Work out the finished part from the listing and answer in its coordinate system (mm). A direction names the side the tool comes from. Coordinates: 2 decimals unless noted, no trailing zeros. Order: outer loops, then holes, each group sorted by start corner. A loop starts at its lowest first (then second) coordinate and runs counter-clockwise, first axis right, second up. Notation, with made-up numbers: (47.25, 72) -> (94.25, 72) arc R21 cw to (94.25, 91) -> close; hole circle Ø1 at (73.25, 22.5). An arc over 180 degrees is marked (long way). Write item = value, one per line. Start each with the question number.
Q1. The part is cut by section A-A, the plane y = 0. Determine the outline of the cut face in (x, z).
Q2. The part is cut by section B-B, the plane z = 0. Determine the outline of the cut face in (x, y).
Q3. Straight lines are drawn through the part: L1, parallel to Z at x = 4.25, y = 0; L2, parallel to X at y = 44, z = 3; L3, parallel to Z at x = 5, y = -44.45. For each, find the intervals that lie inside material, in ascending order. Write a range as from..to.
Q4. Flat-ended cylindrical pins translate along their axes: pin 1 (1 mm diameter, centred on x = 1, y = 7.5, fed in from +Z); pin 2 (5 mm diameter, centred on y = 11, z = 8, fed in from -X); pin 3 (8 mm diameter, centred on y = -16.5, z = -25.5, fed in from -X); pin 4 (1.9 mm diameter, centred on y = 0, z = 44.45, fed in from -X). Find the tip coordinate at first contact, or state that the pin passes through.
Q5. Which of the six approach directions +Z, -Z, +X, -X, +Y, -Y give full straight-line access (tool end or side, diameter ignored) to faces 4 (the cylindrical face through (-7.764, 2.477, -11.155)), 5 (the cylindrical face through (6.26, 0.34, 42.9))?
Q6. The part is cut by section C-C, the plane x = 2. Count the separate pieces of the cut face and the enclosed holes in it, plus the area to 3 significant figures.
Q7. The part is cut by section D-D, the plane y = -44.45. Determine the outline of the cut face in (x, z).
Q8. For a pull along Y with two mould halves and no side action, classify faces 1 (the cylindrical face through (6.3, -10.5, -47.3)), 2 (the flat face through (-15.748, 0, 0)), 3 (the cylindrical face through (6.261, 46.036, 0.07)) as +Y half, -Y half, draft (parallel to the pull), parting line (faces both ways), or undercut.
```python
from build123d import *

# Parameters (mm, degrees)
F0_R     = 48.449945
F1_DEPTH = 12.7
F2_R     = 11.427041
F3_DEPTH = 15.748
F4_R     = 1.5875
F4_R_2   = 1.71099
F5_DEPTH = 12.7


with BuildPart() as f1:
    # F0 (on Right) → F1 (new body)
    with BuildSketch(Plane.YZ):
        Circle(F0_R)
    extrude(amount=F1_DEPTH)

    # F2 (on face) → F3 (join)
    with BuildSketch(Plane(origin=(0, 0, 0), x_dir=(0, -1, 0), z_dir=(-1, 0, 0))):
        Circle(F2_R)
    extrude(amount=F3_DEPTH)

    # F4 (on face) → F5 (cut)
    with BuildSketch(Plane(origin=(0, 0, 0), x_dir=(0, -1, 0), z_dir=(-1, 0, 0))):
        with Locations((0, 44.45)):
            Circle(F4_R)
        with Locations((0, -44.45)):
            Circle(F4_R_2)
        with Locations((44.45, 0)):
            Circle(F4_R)
        with Locations((-44.45, 0)):
            Circle(F4_R)
    extrude(amount=-F5_DEPTH, mode=Mode.SUBTRACT)


solid = f1.part
```
Model answer:
q1.outline = (-15.75, -11.43) -> (0, -11.43) -> (0, -42.74) -> (12.7, -42.74) -> (12.7, 42.86) -> (0, 42.86) -> (0, 11.43) -> (-15.75, 11.43) -> close; (0, -48.45) -> (12.7, -48.45) -> (12.7, -46.16) -> (0, -46.16) -> close; (0, 46.04) -> (12.7, 46.04) -> (12.7, 48.45) -> (0, 48.45) -> close
q2.outline = (-15.75, -11.43) -> (0, -11.43) -> (0, -42.86) -> (12.7, -42.86) -> (12.7, 42.86) -> (0, 42.86) -> (0, 11.43) -> (-15.75, 11.43) -> close; (0, -48.45) -> (12.7, -48.45) -> (12.7, -46.04) -> (0, -46.04) -> close; (0, 46.04) -> (12.7, 46.04) -> (12.7, 48.45) -> (0, 48.45) -> close
q3.L1 = -48.45..-46.16, -42.74..42.86, 46.04..48.45
q3.L2 = 0..12.7
q3.L3 = -19.28..-1.59, 1.59..19.28
q4.pin_1 = 47.94
q4.pin_2 = -15.75
q4.pin_3 = 0
q4.pin_4 = through
q5.face_4 = -X
q5.face_5 = +X, -X
q6.separate_pieces = 1
q6.enclosed_holes = 4
q6.area = 7,340 mm2
q7.outline = (0, -19.28) -> (12.7, -19.28) -> (12.7, -1.59) -> (0, -1.59) -> close; (0, 1.59) -> (12.7, 1.59) -> (12.7, 19.28) -> (0, 19.28) -> close
q8.face_1 = parting line
q8.face_2 = draft
q8.face_3 = undercut
